Design review of the part built by this model. Coordinates are the model's own, in mm. Face numbers are marked on the shaded views. A direction names the side the tool comes from. Coordinates: 2 decimals unless noted, no trailing zeros. Write each loop counter-clockwise with the first axis right and the second up, starting at its lowest first coordinate (ties: lowest second). Pieces come first, ordered by that corner, then holes.
Q1. For L1, parallel to Z at x = -24, y = 6; L2, parallel to Z at x = 8, y = 7.75; L3, parallel to X at y = 4, z = 4, list the stretches that pass through material, from the lowest coordinate up.
Q2. Take a section at C-C, the plane y = 7.5. Write out the cut boundary in (x, z), plus the area to 3 significant figures.
Q3. For the marked faces 1 and 2, list the 3-axis set-ups (+Z, -Z, +X, -X, +Y, -Y) from which the entire face can be reached by the end or side of a thin tool; tool diameter is ignored.
Q4. For pin 1 Ø1 at (y, z) = (1.5, 6) entering from -X; pin 2 Ø3 at (y, z) = (2, 3.5) entering from -X; pin 3 Ø1.5 at (y, z) = (6, 3.5) entering from -X, all flat-tipped, find the tip position at first contact; note any pin that passes through.
Q5. The part is to be moulded in two halves that separate along Z. For the marked faces 3, 4, 5 and 6, say which applies: released by +Z, released by -Z, zero draft, split by the parting line, or undercut.
Q6. Take a section at A-A, the plane z = 0. Write out the cut boundary in (x, y).
Q7. Take a section at B-B, the plane x = -11.5. Write out the cut boundary in (y, z).
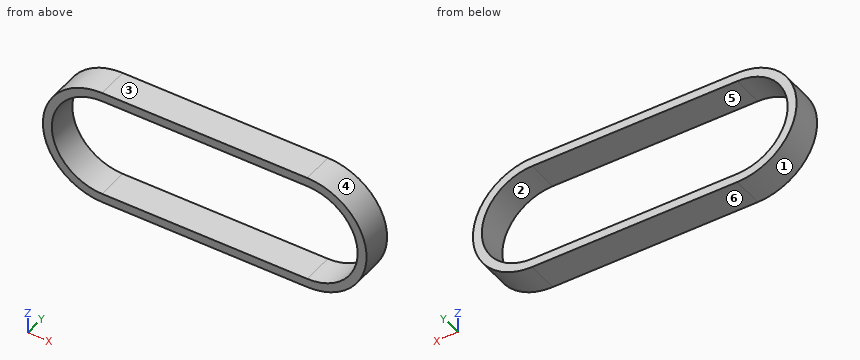
Autodesk Inventor part; units mm, degrees
ref_plane "YZ Plane" through (0, 0, 0) normal (1, 0, 0) x (0, 1, 0)
ref_plane "XZ Plane" through (0, 0, 0) normal (0, 1, 0) x (-1, 0, 0)
ref_plane "XY Plane" through (0, 0, 0) normal (0, 0, 1) x (1, 0, 0)
sketch "Sketch1" plane through (0, 0, 0) normal (0, 1, 0) x (-1, 0, 0)
  circle A0 centre (0, 0) radius 14.3256 construction
  line L0 (0, 0) -> (58.3628, 0) construction
  circle A1 centre (58.3628, 0) radius 14.3256 construction
  line L1 (58.3628, 14.3256) -> (0, 14.3256)
  line L2 (58.3628, -14.3256) -> (0, -14.3256)
  arc A2 (58.3628, -14.3256) -> (58.3628, 14.3256) centre (58.3628, 0) ccw
  arc A3 (0, 14.3256) -> (0, -14.3256) centre (0, 0) ccw
  line L3 (0, 16.8656) -> (58.3628, 16.8656)
  arc A4 (58.3628, -16.8656) -> (58.3628, 16.8656) centre (58.3628, 0) ccw
  line L4 (58.3628, -16.8656) -> (0, -16.8656)
  arc A5 (0, 16.8656) -> (0, -16.8656) centre (0, 0) ccw
  dimension "d0" = 28.6512
  dimension "d1" = 58.3628
  dimension "d2" = 28.6512
  dimension "d3" = 2.54
extrude "Extrusion1" add sketch "Sketch1" along normal blind 8.9916
properties part number "INTK_013_Belt5" material "Rubber, Silicone"
Responses:
1. L1: z = -16.87 to -14.33, 14.33 to 16.87
1. L2: z = -14.85 to -11.88, 11.88 to 14.85
1. L3: x = -74.75 to -72.12, 13.76 to 16.38
2. outline: (-58.36, -16.87) - (0, -16.87) arc R16.87 ccw to (0, 16.87) - (-58.36, 16.87) arc R16.87 ccw to start; hole (-58.36, -14.33) - (0, -14.33) arc R14.33 ccw to (0, 14.33) - (-58.36, 14.33) arc R14.33 ccw to start
2. area: 545 mm2
3. face 1: -X, +Y, -Y
3. face 2: +Y, -Y
4. pin 1: stops at x = -74.31
4. pin 2: stops at x = -75.11
4. pin 3: stops at x = -75
5. face 3: released by +Z
5. face 4: split by the parting line
5. face 5: undercut
5. face 6: released by -Z
6. outline: (-75.23, 0) - (-72.69, 0) - (-72.69, 8.99) - (-75.23, 8.99) - close; (14.33, 0) - (16.87, 0) - (16.87, 8.99) - (14.33, 8.99) - close
7. outline: (0, -16.87) - (8.99, -16.87) - (8.99, -14.33) - (0, -14.33) - close; (0, 14.33) - (8.99, 14.33) - (8.99, 16.87) - (0, 16.87) - close
